Could you check a few things on this model? Use its own coordinates, in mm. A direction names the side the tool comes from. Round coordinates to 2 decimals unless told otherwise and drop trailing zeros. Write each loop counter-clockwise with the first axis right and the second up, starting at its lowest first coordinate (ties: lowest second). Pieces come first, ordered by that corner, then holes. Notation, with made-up numbers: M 64,74.5 L 78,74.5 A13 ccw 78,83.5 Z; hole C 69,0 d10. An arc over 180 degrees is marked long. One line per item, written item: value. Start each with the question number.
(1) If I drill on L1, parallel to Y at x = -1, z = -8; L2, parallel to X at y = 2.95, z = 0; L3, parallel to Z at x = 1.5, y = 3.55, over which ranges is the centre line in solid material (lowest first)?
(2) Thinking about a two-plate mould opening in X: for faces 1 (the face through (0, 0.5, -13)), 2 (the face through (-1.245, 1.972, 3.002)), 3 (the face through (0, 0, 0)), which applies, released by +X, released by -X, zero draft, split by the parting line, or undercut?
(3) I want a section at B-B on y = 0.3. Count the separate pieces of the cut face and the enclosed holes in it, and give its area (3 significant figures).
(4) I want a section at A-A on z = -10.5. Please give me the cut outline in (x, y), and give its area (3 significant figures).
(5) I want a section at C-C on x = 1. Please give me the cut outline in (y, z).
(6) I'm going to push flat-ended pins straight in: pin 1 Ø2 at (x, y) = (1.5, 3.5) entering from -Z; pin 2 Ø1.5 at (x, y) = (-2, 2) entering from +Z; pin 3 Ø2 at (x, z) = (-2, -8) entering from +Y. Where does each tip first touch, or does it pass through?
(7) Which directions (+Z, -Z, +X, -X, +Y, -Y) give clear straight access to the entire face, cutting with the end or side of a thin tool? Please do faces 4 (the face through (0.676, 2.479, 2.146)), 5 (the face through (2.007, 0.493, -8.448)).
(8) I want a section at D-D on z = 8.5. Please give me the cut outline in (x, y), and give its area (3 significant figures).
```python
from build123d import *

# Parameters (mm, degrees)
SKETCH_1_R      = 3.25
SKETCH_1_R_2    = 2.25
EXTRUDE_1_DEPTH = 4
SKETCH_1_3_R    = 2.25
EXTRUDE_2_DEPTH = 1
SKETCH_1_4_R    = 0.5
EXTRUDE_3_DEPTH = 1
SKETCH_1_5_R    = 0.5
EXTRUDE_4_DEPTH = 1


with BuildPart() as part:
    # Sketch 1 → Extrude 1 (new body)
    with BuildSketch(Plane(origin=(0, 0, 0), x_dir=(1, 0, 0), z_dir=(0, 1, 0))):
        with Locations(Location((0, 0, 0), (0, 0, 270))):
            Circle(SKETCH_1_R)
        with Locations(Location((0, 0, 0), (0, 0, 270))):
            Circle(SKETCH_1_R_2, mode=Mode.SUBTRACT)
    extrude(amount=EXTRUDE_1_DEPTH)

    # Sketch 1_3 → Extrude 2 (add)
    with BuildSketch(Plane(origin=(0, 0, 0), x_dir=(1, 0, 0), z_dir=(0, 1, 0))):
        with Locations(Location((0, 0, 0), (0, 0, 270))):
            Circle(SKETCH_1_3_R)
    extrude(amount=EXTRUDE_2_DEPTH)

    # Sketch 1_4 → Extrude 3 (add)
    with BuildSketch(Plane(origin=(0, 0, 0), x_dir=(1, 0, 0), z_dir=(0, 1, 0))):
        with BuildLine():
            ThreePointArc((1.5, 15), (0, 15.677124344), (-1.5, 15))
            Line((-1.5, 15), (-2.5, 2.076655966))
            ThreePointArc((-2.5, 2.076655966), (0, 3.25), (2.5, 2.076655966))
            Line((2.5, 2.076655966), (1.5, 15))
        make_face()
        with Locations(Location((0, 4.5, 0), (0, 0, 270))):
            Circle(SKETCH_1_4_R, mode=Mode.SUBTRACT)
        with Locations(Location((0, 6.5, 0), (0, 0, 270))):
            Circle(SKETCH_1_4_R, mode=Mode.SUBTRACT)
        with Locations(Location((0, 8.5, 0), (0, 0, 270))):
            Circle(SKETCH_1_4_R, mode=Mode.SUBTRACT)
        with Locations(Location((0, 10.5, 0), (0, 0, 270))):
            Circle(SKETCH_1_4_R, mode=Mode.SUBTRACT)
        with Locations(Location((0, 12.5, 0), (0, 0, 270))):
            Circle(SKETCH_1_4_R, mode=Mode.SUBTRACT)
        with Locations(Location((0, 14.5, 0), (0, 0, 270))):
            Circle(SKETCH_1_4_R, mode=Mode.SUBTRACT)
    extrude(amount=EXTRUDE_3_DEPTH)

    # Sketch 1_5 → Extrude 4 (add)
    with BuildSketch(Plane(origin=(0, 0, 0), x_dir=(1, 0, 0), z_dir=(0, 1, 0))):
        with BuildLine():
            ThreePointArc((2.5, -2.076655966), (0, -3.25), (-2.5, -2.076655966))
            Line((-2.5, -2.076655966), (-1.5, -15))
            ThreePointArc((-1.5, -15), (0, -15.677124344), (1.5, -15))
            Line((1.5, -15), (2.5, -2.076655966))
        make_face()
        with Locations(Location((0, -14.5, 0), (0, 0, 270))):
            Circle(SKETCH_1_5_R, mode=Mode.SUBTRACT)
        with Locations(Location((0, -12.5, 0), (0, 0, 270))):
            Circle(SKETCH_1_5_R, mode=Mode.SUBTRACT)
        with Locations(Location((0, -10.5, 0), (0, 0, 270))):
            Circle(SKETCH_1_5_R, mode=Mode.SUBTRACT)
        with Locations(Location((0, -8.5, 0), (0, 0, 270))):
            Circle(SKETCH_1_5_R, mode=Mode.SUBTRACT)
        with Locations(Location((0, -6.5, 0), (0, 0, 270))):
            Circle(SKETCH_1_5_R, mode=Mode.SUBTRACT)
        with Locations(Location((0, -4.5, 0), (0, 0, 270))):
            Circle(SKETCH_1_5_R, mode=Mode.SUBTRACT)
    extrude(amount=EXTRUDE_4_DEPTH)


solid = part.part
```
Found:
1. L1: y = 0 to 1
1. L2: x = -3.25 to -2.25, 2.25 to 3.25
1. L3: z = -2.88 to -1.68, 1.68 to 2.88
2. face 1: undercut
2. face 2: split by the parting line
2. face 3: zero draft
3. separate pieces: 1
3. enclosed holes: 12
3. area: 122 mm²
4. outline: M -1.85,0 L -0.5,0 L -0.5,1 L -1.85,1 Z; M 0.5,0 L 1.85,0 L 1.85,1 L 0.5,1 Z
4. area: 2.70 mm²
5. outline: M 0,-15.41 L 1,-15.41 L 1,-3.09 L 4,-3.09 L 4,-2.02 L 1,-2.02 L 1,2.02 L 4,2.02 L 4,3.09 L 1,3.09 L 1,15.41 L 0,15.41 Z
6. pin 1: stops at z = -3.21
6. pin 2: stops at z = 3
6. pin 3: stops at y = 1
7. face 4: +Y
7. face 5: -Z, +X, +Y, -Y
8. outline: M -2,0 L -0.5,0 L -0.5,1 L -2,1 Z; M 0.5,0 L 2,0 L 2,1 L 0.5,1 Z
8. area: 3.01 mm²
